The model under review builds one solid part; all positions refer to its coordinate system, in mm. A direction names the side the tool comes from. Round coordinates to 2 decimals unless told otherwise and drop trailing zeros. Write each loop counter-clockwise with the first axis right and the second up, starting at its lowest first coordinate (ties: lowest second). Pieces come first, ordered by that corner, then holes.
Item 1: Add section A-A (y = -7). Give the boundary of the cut face in (x, z) (3 decimals), plus the area to 3 significant figures.
Item 2: To check wall thickness, follow L1, parallel to X at y = 0, z = 5.3; L2, parallel to Y at x = -5.3, z = 5.4; L3, parallel to X at y = -4.3, z = 9. State the ranges of each line that lie inside material, in increasing order.
Item 3: Draft analysis for pull direction Y (two halves, no side actions). For faces 1 (the face through (-3.05, -6.53, 7.27)), 2 (the face through (3.05, 1.73, 14.23)), 3 (the face through (0, -8.3, 4)), state which applies: +Y half, -Y half, draft (parallel to the pull), parting line (faces both ways), or undercut.
Item 4: Clearance check with flat-ended pins moving along their axes: pin 1 Ø3 at (x, z) = (0, 9) entering from -Y; pin 2 Ø2 at (x, y) = (0, 1.5) entering from +Z; pin 3 Ø3.5 at (x, z) = (0.5, 10.5) entering from -Y. State where each tip first meets the part, or that it passes through.
Item 5: Add section C-C (z = 1.5). Give the boundary of the cut face in (x, y), plus the area to 3 significant figures.
Item 6: Add section B-B (x = 0). Give the boundary of the cut face in (y, z).
Item 7: Add section D-D (x = -5.3). Give the boundary of the cut face in (y, z).
Item 8: Machinability: for faces 4 (the face through (-8.3, 0, 8)), 5 (the face through (-6.787, -0.195, 5.087)), 6 (the face through (-7, -1, 4.2)), 7 (the face through (0, -7, 5.493)), 8 (the face through (-3.05, -1.73, 14.23)), which of the approach directions +Z, -Z, +X, -X, +Y, -Y give a long, thin tool a straight path to every point of the face, cutting with its end or side? Answer none if there is none.
```python
from build123d import *

# Parameters (mm, degrees)
CYLINDER002_R           = 1.5
CYLINDER002_DEPTH       = 6
SKETCH003_W             = 5.5
SKETCH003_H             = 6
PAD003_DEPTH            = 1.2
FUSION_PLACEMENT_ANGLE  = 90
PAD002_DEPTH            = 3.5
BODY002_PLACEMENT_ANGLE = 90
PAD001_DEPTH            = 3.5
CYLINDER_R              = 2
CYLINDER_DEPTH          = 16
CYLINDER001_R           = 2
CYLINDER001_DEPTH       = 5.4
BOX_W                   = 16.6
BOX_H                   = 16.6
BOX_DEPTH               = 16


with BuildPart() as cylinder002:
    # Cylinder002 → Cylinder002 (new body)
    with BuildSketch(Plane(origin=(0, 3, -3), x_dir=(1, 0, 0), z_dir=(0, 0, 1))):
        Circle(CYLINDER002_R)
    extrude(amount=CYLINDER002_DEPTH)


with BuildPart() as fusion:
    # Sketch003 → Pad003 (new body, symmetric)
    with BuildSketch(Plane.XY):
        with Locations((0, 3)):
            Rectangle(SKETCH003_W, SKETCH003_H)
    extrude(amount=PAD003_DEPTH, both=True)

    # Fusion: union Cylinder002
    add(cylinder002.part)


with BuildPart() as fusion_1:
    # Fusion placement: moved
    add(fusion.part.moved(Location((-2.3, 0, 3))).rotate(Axis((-2.3, 0, 3), (0, 0, 1)), FUSION_PLACEMENT_ANGLE))


with BuildPart() as nut_body002:
    # Sketch002 → Pad002 (new body)
    with BuildSketch(Plane.XY):
        Polygon((-4.05, 0), (-2.025, -3.507403), (2.025, -3.507403), (4.05, 0), (2.025, 3.507403), (-2.025, 3.507403), align=None)
    extrude(amount=PAD002_DEPTH)


with BuildPart() as nut_body002_1:
    # Body002 placement: moved
    add(nut_body002.part.moved(Location((0, -4.8, 9))).rotate(Axis((0, -4.8, 9), (1, 0, 0)), BODY002_PLACEMENT_ANGLE))


with BuildPart() as nut_body:
    # Sketch001 → Pad001 (new body)
    with BuildSketch(Plane.XY):
        Polygon((-4.05, 0), (-2.025, -3.507403), (2.025, -3.507403), (4.05, 0), (2.025, 3.507403), (-2.025, 3.507403), align=None)
    extrude(amount=PAD001_DEPTH)


with BuildPart() as nut_body_1:
    # Body001 placement: moved
    add(nut_body.part.moved(Location((0, 0, 12.5))))


with BuildPart() as cylinder:
    # Cylinder → Cylinder (new body)
    with BuildSketch(Plane.XY):
        Circle(CYLINDER_R)
    extrude(amount=CYLINDER_DEPTH)


with BuildPart() as fusion001:
    # Cylinder001 → Cylinder001 (new body)
    with BuildSketch(Plane(origin=(0, -8.3, 9), x_dir=(1, 0, 0), z_dir=(0, 1, 0))):
        Circle(CYLINDER001_R)
    extrude(amount=CYLINDER001_DEPTH)

    # Fusion001: union Fusion, nut_body002, nut_body, Cylinder
    add(fusion_1.part)
    add(nut_body002_1.part)
    add(nut_body_1.part)
    add(cylinder.part)


with BuildPart() as cut:
    # Box → Box (new body)
    with BuildSketch(Plane(origin=(-8.3, -8.3, 0), x_dir=(1, 0, 0), z_dir=(0, 0, 1))):
        with Locations((8.3, 8.3)):
            Rectangle(BOX_W, BOX_H)
    extrude(amount=BOX_DEPTH)

    # Cut: cut Fusion001
    add(fusion001.part, mode=Mode.SUBTRACT)


solid = cut.part
```
Numbers:
1. outline: (-8.3, 0) - (8.3, 0) - (8.3, 16) - (-8.3, 16) - close; hole (-4.05, 9) - (-2.025, 5.493) - (2.025, 5.493) - (4.05, 9) - (2.025, 12.507) - (-2.025, 12.507) - close
1. area: 223 mm2
2. L1: x = -8.3 to -6.8, -3.8 to -2, 2 to 8.3
2. L2: y = -8.3 to -1.5, 1.5 to 8.3
2. L3: x = -8.3 to -2, 2 to 8.3
3. face 1: draft
3. face 2: undercut
3. face 3: -Y half
4. pin 1: stops at y = -2.9
4. pin 2: stops at z = 12.5
4. pin 3: stops at y = -4.8
5. outline: (-8.3, -8.3) - (8.3, -8.3) - (8.3, 8.3) - (-8.3, 8.3) - close; hole circle Ø3 at (-5.3, 0); hole circle Ø4 at (0, 0)
5. area: 256 mm2
6. outline: (-8.3, 0) - (-2, 0) - (-2, 12.5) - (-3.51, 12.5) - (-3.51, 16) - (-8.3, 16) - (-8.3, 12.51) - (-4.8, 12.51) - (-4.8, 11) - (-2.9, 11) - (-2.9, 7) - (-4.8, 7) - (-4.8, 5.49) - (-8.3, 5.49) - close; (2, 0) - (8.3, 0) - (8.3, 16) - (3.51, 16) - (3.51, 12.5) - (2, 12.5) - close
7. outline: (-8.3, 0) - (-1.5, 0) - (-1.5, 1.8) - (-2.75, 1.8) - (-2.75, 4.2) - (-1.5, 4.2) - (-1.5, 6) - (1.5, 6) - (1.5, 4.2) - (2.75, 4.2) - (2.75, 1.8) - (1.5, 1.8) - (1.5, 0) - (8.3, 0) - (8.3, 16) - (-8.3, 16) - close
8. face 4: +Z, -Z, -X, +Y, -Y
8. face 5: -Z
8. face 6: -X
8. face 7: -Y
8. face 8: +Z
